Input: part model. Units: mm. Frame: model coordinates. Face numbers are marked on the shaded views. Coordinates: 2 decimals unless noted, no trailing zeros. Order: outer loops, then holes, each group sorted by start corner. A loop starts at its lowest first (then second) coordinate and runs counter-clockwise, first axis right, second up. Notation, with made-up numbers: (-36, 53) - (23, 53) arc R25 cw to (23, 73) - close; hole circle Ø3 at (61.25, 41). An arc over 180 degrees is marked (long way). One line per question, with ' | ' between items. Start each with the question number.
```python
from build123d import *

# Parameters (mm, degrees)
F2_DEPTH = 12.7
F3_W     = 7
F3_H     = 4.492721
F3_W_2   = 5.5
F3_H_2   = 1.6
F4_DEPTH = 12.7


with BuildPart() as f1:
    # F0 (on Front) → F1 (revolve)
    with BuildSketch(Plane.XZ):
        with BuildLine():
            ThreePointArc((-1, 0), (0, 1), (1, 0))
            Line((1, 0), (53.45, 0))
            ThreePointArc((53.45, 0), (54, 0.55), (54.55, 0))
            Line((54.55, 0), (57, 0))
            Line((57, 0), (57, 1.5))
            Line((57, 1.5), (56, 2.5))
            Line((56, 2.5), (50.5, 2.5))
            Line((50.5, 2.5), (49.5, 1.5))
            Line((49.5, 1.5), (5, 1.5))
            Line((5, 1.5), (4, 2.5))
            Line((4, 2.5), (-4, 2.5))
            Line((-4, 2.5), (-5, 1.5))
            Line((-5, 1.5), (-5, 0))
            Line((-5, 0), (-1, 0))
        make_face()
        with BuildLine():
            ThreePointArc((-1, 0), (0, -1), (1, 0))
            Line((1, 0), (-1, 0))
        make_face()
        with BuildLine():
            Line((54.55, 0), (53.45, 0))
            ThreePointArc((53.45, 0), (54, -0.55), (54.55, 0))
        make_face()
    revolve(axis=Axis((26, 0, 0), (1, 0, 0)))

    # F0 (on Front) → F2 (cut, symmetric)
    with BuildSketch(Plane.XZ):
        with BuildLine():
            Line((-1, 0), (1, 0))
            ThreePointArc((1, 0), (0, 1), (-1, 0))
        make_face()
        with BuildLine():
            ThreePointArc((-1, 0), (0, -1), (1, 0))
            Line((1, 0), (-1, 0))
        make_face()
        with BuildLine():
            ThreePointArc((54.55, 0), (54, 0.55), (53.45, 0))
            Line((53.45, 0), (54.55, 0))
        make_face()
        with BuildLine():
            Line((54.55, 0), (53.45, 0))
            ThreePointArc((53.45, 0), (54, -0.55), (54.55, 0))
        make_face()
    extrude(amount=F2_DEPTH, both=True, mode=Mode.SUBTRACT)

    # F3 (on Top) → F4 (cut, symmetric)
    with BuildSketch(Plane.XY):
        with Locations((0, 2.24636)):
            Rectangle(F3_W, F3_H)
        with Locations((54.25, 0)):
            Rectangle(F3_W_2, F3_H_2)
    extrude(amount=F4_DEPTH, both=True, mode=Mode.SUBTRACT)


solid = f1.part
```
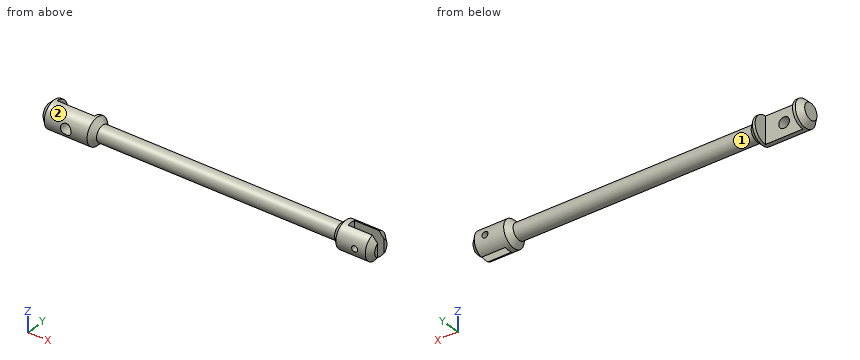
(1) Section A-A (x = 54). Output: boundary loops of the cut face in (y, z).
(2) Draft query along X for the marked faces 1 and 2. Return one class per face: +X half, -X half, draft (parallel to the pull), parting line (faces both ways), or undercut.
(3) Section C-C (x = 0). Output: boundary loops of the cut face in (y, z), then the cut area to 3 significant figures.
(4) Section D-D (x = 43). Output: boundary loops of the cut face in (y, z).
(5) Pin query (flat end, axial travel): pin 1 (1 mm diameter, centred on x = 20, z = -0.5, fed in from +Y); pin 2 (0.8 mm diameter, centred on y = 0, z = 0.5, fed in from +X); pin 3 (1 mm diameter, centred on x = 2.5, y = -1.5, fed in from +Z). Return the tip coordinate at first contact, or that it passes through.
(6) Section B-B (z = 0). State how many separate pieces and enclosed holes the cut face has, then the cut area to 3 significant figures.
(7) Material intervals for line 1 along X through (y, z) = (-1.25, 0.4); line 2 along Z through (x, y) = (54, 2); line 3 along X through (y, z) = (2.1, 1), sorted ascending. Write a range as from..to.
Worked answers:
1) outline: (-2.44, -0.55) arc R2.5 ccw to (-0.8, -2.37) - (-0.8, -0.55) - close; (-2.44, 0.55) - (-0.8, 0.55) - (-0.8, 2.37) arc R2.5 ccw to start; (0.8, -2.37) arc R2.5 ccw to (2.44, -0.55) - (0.8, -0.55) - close; (0.8, 0.55) - (2.44, 0.55) arc R2.5 ccw to (0.8, 2.37) - close
2) face 1: undercut | face 2: draft
3) outline: (-2.29, -1) arc R2.5 ccw to (0, -2.5) - (0, -1) - close; (-2.29, 1) - (0, 1) - (0, 2.5) arc R2.5 ccw to start | area: 4.95 mm²
4) outline: circle Ø3 at (0, 0)
5) pin 1: stops at y = 1.5 | pin 2: stops at x = 51.5 | pin 3: stops at z = 2.29
6) separate pieces: 4 | enclosed holes: 0 | area: 182 mm²
7) line 1: x = -5..-0.92, 0.92..53.62, 54.38..57 | line 2: z = -1.5..-0.55, 0.55..1.5 | line 3: x = -4.17..-3.5, 3.5..4.17, 50.33..56.17
